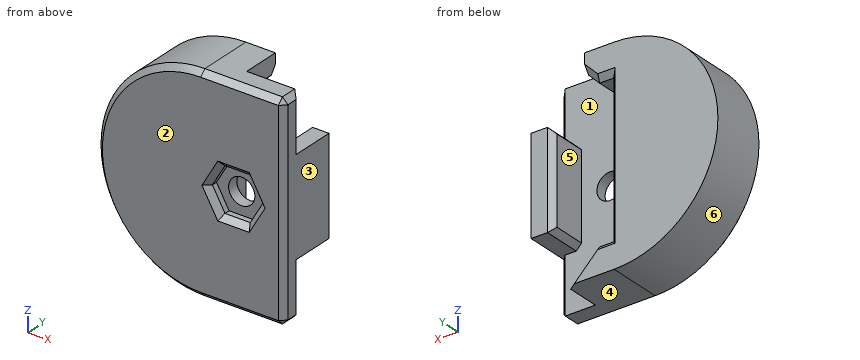
from build123d import *

# Parameters (mm, degrees)
SKETCH1_R           = 1.2
BOSS_EXTRUDE1_DEPTH = 2
SKETCH2_W           = 2
SKETCH2_H           = 8.8
BOSS_EXTRUDE2_DEPTH = 3.5
CUT_EXTRUDE1_DEPTH  = 1
CHAMFER1_SIZE       = 0.5


with BuildPart() as part:
    # Sketch1 → Boss-Extrude1 (new body)
    with BuildSketch(Plane(origin=(0, 0, 0), x_dir=(1, 0, 0), z_dir=(0, 1, 0))):
        with BuildLine():
            Line((4.6, -9.5), (4.6, 9.5))
            Line((4.6, 9.5), (-3, 9.5))
            ThreePointArc((-3, 9.5), (-12.5, 0), (-3, -9.5))
            Line((-3, -9.5), (4.6, -9.5))
        make_face()
        with Locations(Location((0, 0, 0), (0, 0, 270))):
            Circle(SKETCH1_R, mode=Mode.SUBTRACT)
    extrude(amount=BOSS_EXTRUDE1_DEPTH)

    # Sketch2 → Boss-Extrude2 (add)
    with BuildSketch(Plane(origin=(0, 2, 0), x_dir=(1, 0, 0), z_dir=(0, 1, 0))):
        with Locations((3.6, 0)):
            Rectangle(SKETCH2_W, SKETCH2_H)
        with BuildLine():
            Line((-2.6, -6.85), (-2.6, 6.85))
            Line((-2.6, 6.85), (-1.3, 6.85))
            Line((-1.3, 6.85), (1.35, 9.5))
            Line((1.35, 9.5), (-3, 9.5))
            ThreePointArc((-3, 9.5), (-12.5, 0), (-3, -9.5))
            Line((-3, -9.5), (-0.3, -9.5))
            Line((-0.3, -9.5), (-0.3, -7.85))
            Line((-0.3, -7.85), (-1.3, -6.85))
            Line((-1.3, -6.85), (-2.6, -6.85))
        make_face()
    extrude(amount=BOSS_EXTRUDE2_DEPTH)

    # Sketch3 → Cut-Extrude1 (cut)
    with BuildSketch(Plane.XZ):
        Polygon((-2.309401077, 0), (-1.154700538, -2), (1.154700538, -2), (2.309401077, 0), (1.154700538, 2), (-1.154700538, 2), align=None)
    extrude(amount=-CUT_EXTRUDE1_DEPTH, mode=Mode.SUBTRACT)

    # Chamfer1
    chamfer1_edges = [part.edges().sort_by_distance(p)[0] for p in [
        (4.6, 2, 6.95),
        (-0.8, 5.5, 7.35),
        (-1.95, 5.5, 6.85),
        (-2.6, 5.5, 0),
        (-1.95, 5.5, -6.85),
        (0.025, 5.5, -8.175),
        (4.6, 2, -6.95),
        (2.6, 3.75, -4.4),
        (2.6, 3.75, 4.4),
        (2.6, 5.5, 0),
        (4.6, 0, 0),
        (0.8, 0, 9.5),
        (-12.5, 0, 0),
        (0.8, 0, -9.5),
        (-1.732050808, 0, 1),
        (-1.732050808, 0, -1),
        (0, 0, -2),
        (1.732050808, 0, -1),
        (1.732050808, 0, 1),
        (0, 0, 2),
        (4.6, 1, -9.5),
        (4.6, 1, 9.5),
    ]]
    chamfer(chamfer1_edges, length=CHAMFER1_SIZE)


solid = part.part
Can you work these out from the model? Positions are in its coordinate system, mm. Face numbers are marked on the shaded views. A direction names the side the tool comes from. Give positions to 0.01 mm unless a question says otherwise; leave off trailing zeros. Write each loop counter-clockwise with the first axis right and the second up, starting at its lowest first coordinate (ties: lowest second). Pieces come first, ordered by that corner, then holes. Notation, with made-up numbers: M 76.25,82.5 L 119.25,82.5 A14 cw 119.25,91.5 Z; hole C 54.25,-20.5 d1. An arc over 180 degrees is marked long. Answer in a Markdown table with one row per item. Add a question column.
Item 1: Please list where these lines run through material, in increasing order: L1, parallel to Z at x = 0, y = 1.75; L2, parallel to X at y = 1.6, z = 0; L3, parallel to Y at x = 2, z = 5.5.
Item 2: Imagine slicing it at B-B, the plane x = 0. Write out the boundary of the cut face in (y, z).
Item 3: On a 3-axis mill with a long thin cutter (end or side, diameter ignored), from which of +Z, -Z, +X, -X, +Y, -Y can I reach the whole of each face in a straight line? I mean the marked faces 1 and 2. Say none if no direction works.
Item 4: For pin 1 Ø1.5 at (x, y) = (-9.5, 4.5) entering from -Z; pin 2 Ø1 at (y, z) = (3.5, -2) entering from -X; pin 3 Ø3.5 at (x, z) = (-0.5, 3.5) entering from +Y; pin 4 Ø1.2 at (x, z) = (0, 0.5) entering from -Y, each with a flat end and sliding along its axis, tell me the tip position at first contact or that it passes through.
Item 5: Imagine slicing it at C-C, the plane y = 4.2. Write out the boundary of the cut face in (x, z).
Item 6: Imagine slicing it at A-A, the plane y = 1.25. Write out the boundary of the cut face in (x, z).
Item 7: We'd pull the mould along X, two halves only. Please class the marked faces 3, 4, 5 and 6: released by +X, released by -X, zero draft, split by the parting line, or undercut.
Evaluation:
| question | item | result |
|---|---|---|
| 1 | L1 | z = -9.5 to -1.2, 1.2 to 9.5 |
| 1 | L2 | x = -12.5 to -1.2, 1.2 to 4.6 |
| 1 | L3 | y = 0 to 2 |
| 2 | outline | M 0,-9 L 0.5,-9.5 L 5.5,-9.5 L 5.5,-8.86 L 5,-8.15 L 2,-8.15 L 2,-1.2 L 1,-1.2 L 1,-2 L 0.5,-2 L 0,-2.5 Z; M 0,2.5 L 0.5,2 L 1,2 L 1,1.2 L 2,1.2 L 2,9.5 L 0.5,9.5 L 0,9 Z |
| 3 | face 1 | +Y |
| 3 | face 2 | +Z, -Z, +X, -X, -Y |
| 4 | pin 1 | stops at z = -7.56 |
| 4 | pin 2 | stops at x = -12.38 |
| 4 | pin 3 | stops at y = 2 |
| 4 | pin 4 | passes through |
| 5 | outline | M -3,-9.5 L 1.35,-9.5 L -1.3,-6.85 L -2.6,-6.85 L -2.6,6.85 L -1.3,6.85 L -0.3,7.85 L -0.3,9.5 L -3,9.5 A9.5 ccw Z; M 2.6,-3.9 L 3.1,-4.4 L 4.6,-4.4 L 4.6,4.4 L 3.1,4.4 L 2.6,3.9 Z |
| 6 | outline | M -3,-9.5 L 4.1,-9.5 L 4.6,-9 L 4.6,9 L 4.1,9.5 L -3,9.5 A9.5 ccw Z; hole C 0,0 d2.4 |
| 7 | face 3 | released by +X |
| 7 | face 4 | zero draft |
| 7 | face 5 | undercut |
| 7 | face 6 | released by -X |
